from build123d import *

# Parameters (mm, degrees)
YAW_PLATFORM_START                         = 72
YAW_PLATFORM_PROFILE_R                     = 44
YAW_PLATFORM_DEPTH                         = 5
PRINTED_HOLLOW_YAW_SPINDLE_START           = 43
PRINTED_HOLLOW_YAW_SPINDLE_PROFILE_R       = 3.95
PRINTED_HOLLOW_YAW_SPINDLE_PROFILE_R_2     = 1.75
PRINTED_HOLLOW_YAW_SPINDLE_DEPTH           = 29
INNER_RACE_LOAD_SHOULDER_START             = 70
INNER_RACE_LOAD_SHOULDER_PROFILE_R         = 6
INNER_RACE_LOAD_SHOULDER_PROFILE_R_2       = 1.75
INNER_RACE_LOAD_SHOULDER_DEPTH             = 2
D_FLAT_ON_SPINDLE_END_START                = 43
D_FLAT_DRIVE_KEY_PROFILE_W                 = 3
D_FLAT_DRIVE_KEY_PROFILE_H                 = 10
D_FLAT_ON_SPINDLE_END_DEPTH                = 5
SHOULDER_MOUNT_PLATE_PROFILE_W             = 87
SHOULDER_MOUNT_PLATE_PROFILE_H             = 68
SHOULDER_MOUNT_PLATE_DEPTH                 = 4
MG996_BODY_WINDOW_START                    = -5
MG996_BODY_WINDOW_PROFILE_W                = 41.7
MG996_BODY_WINDOW_PROFILE_H                = 20.7
MG996_BODY_WINDOW_DEPTH                    = 162.869372409
MG996_TAB_MOUNTS_START                     = -50
MG996_TAB_MOUNTS_PROFILE_R                 = 1.9
MG996_TAB_MOUNTS_DEPTH                     = 207.869372409
PASSIVE_SHOULDER_STANDOFFS_START           = -50
PASSIVE_SHOULDER_STANDOFFS_PROFILE_R       = 1.6
PASSIVE_SHOULDER_STANDOFFS_DEPTH           = 207.869372409
UPRIGHT_RIB_START                          = -8
UPRIGHT_RIB_PROFILE_W                      = 7
UPRIGHT_RIB_PROFILE_H                      = 31
UPRIGHT_RIB_DEPTH                          = 12
YAW_POSITIVE_RETENTION_CROSSBOLT_START     = -10
YAW_POSITIVE_RETENTION_CROSSBOLT_PROFILE_R = 1.1
YAW_POSITIVE_RETENTION_CROSSBOLT_DEPTH     = 167.869372409


with BuildPart() as part:
    # Yaw_platform_profile → Yaw_platform (new body)
    with BuildSketch(Plane(origin=(0, 0, 0), x_dir=(1, 0, 0), z_dir=(0, 1, 0)).offset(YAW_PLATFORM_START)):
        with Locations(Location((0, 0, 0), (0, 0, 270))):
            Circle(YAW_PLATFORM_PROFILE_R)
    extrude(amount=YAW_PLATFORM_DEPTH)

    # Printed_hollow_yaw_spindle_profile → Printed_hollow_yaw_spindle (add)
    with BuildSketch(Plane(origin=(0, 0, 0), x_dir=(1, 0, 0), z_dir=(0, 1, 0)).offset(PRINTED_HOLLOW_YAW_SPINDLE_START)):
        with Locations(Location((0, 0, 0), (0, 0, 90))):
            Circle(PRINTED_HOLLOW_YAW_SPINDLE_PROFILE_R)
        with Locations(Location((0, 0, 0), (0, 0, 90))):
            Circle(PRINTED_HOLLOW_YAW_SPINDLE_PROFILE_R_2, mode=Mode.SUBTRACT)
    extrude(amount=PRINTED_HOLLOW_YAW_SPINDLE_DEPTH)

    # Inner_race_load_shoulder_profile → Inner_race_load_shoulder (add)
    with BuildSketch(Plane(origin=(0, 0, 0), x_dir=(1, 0, 0), z_dir=(0, 1, 0)).offset(INNER_RACE_LOAD_SHOULDER_START)):
        with Locations(Location((0, 0, 0), (0, 0, 270))):
            Circle(INNER_RACE_LOAD_SHOULDER_PROFILE_R)
        with Locations(Location((0, 0, 0), (0, 0, 90))):
            Circle(INNER_RACE_LOAD_SHOULDER_PROFILE_R_2, mode=Mode.SUBTRACT)
    extrude(amount=INNER_RACE_LOAD_SHOULDER_DEPTH)

    # D_flat_drive_key_profile → D_flat_on_spindle_end (cut)
    with BuildSketch(Plane(origin=(0, 0, 0), x_dir=(1, 0, 0), z_dir=(0, 1, 0)).offset(D_FLAT_ON_SPINDLE_END_START)):
        with Locations((4.5, 0)):
            Rectangle(D_FLAT_DRIVE_KEY_PROFILE_W, D_FLAT_DRIVE_KEY_PROFILE_H)
    extrude(amount=D_FLAT_ON_SPINDLE_END_DEPTH, mode=Mode.SUBTRACT)

    # Shoulder_mount_plate_profile → Shoulder_mount_plate (add)
    with BuildSketch(Plane.XY):
        with Locations((-0.5, 110)):
            Rectangle(SHOULDER_MOUNT_PLATE_PROFILE_W, SHOULDER_MOUNT_PLATE_PROFILE_H)
    extrude(amount=SHOULDER_MOUNT_PLATE_DEPTH)

    # MG996_body_window_profile → MG996_body_window (cut, through all)
    with BuildSketch(Plane.XY.offset(MG996_BODY_WINDOW_START)):
        with Locations((10.35, 122)):
            Rectangle(MG996_BODY_WINDOW_PROFILE_W, MG996_BODY_WINDOW_PROFILE_H)
    extrude(amount=MG996_BODY_WINDOW_DEPTH, mode=Mode.SUBTRACT)

    # MG996_tab_mounts_profile → MG996_tab_mounts (cut, through all)
    with BuildSketch(Plane.XY.offset(MG996_TAB_MOUNTS_START)):
        with Locations(Location((-13, 117, 0), (0, 0, 180))):
            Circle(MG996_TAB_MOUNTS_PROFILE_R)
        with Locations(Location((-13, 127, 0), (0, 0, 180))):
            Circle(MG996_TAB_MOUNTS_PROFILE_R)
        with Locations(Location((34, 117, 0), (0, 0, 180))):
            Circle(MG996_TAB_MOUNTS_PROFILE_R)
        with Locations(Location((34, 127, 0), (0, 0, 180))):
            Circle(MG996_TAB_MOUNTS_PROFILE_R)
    extrude(amount=MG996_TAB_MOUNTS_DEPTH, mode=Mode.SUBTRACT)

    # Passive_shoulder_standoffs_profile → Passive_shoulder_standoffs (cut, through all)
    with BuildSketch(Plane.XY.offset(PASSIVE_SHOULDER_STANDOFFS_START)):
        with Locations(Location((-36, 104, 0), (0, 0, 180))):
            Circle(PASSIVE_SHOULDER_STANDOFFS_PROFILE_R)
        with Locations(Location((-36, 140, 0), (0, 0, 180))):
            Circle(PASSIVE_SHOULDER_STANDOFFS_PROFILE_R)
    extrude(amount=PASSIVE_SHOULDER_STANDOFFS_DEPTH, mode=Mode.SUBTRACT)

    # Upright_rib_profile → Upright_rib (add)
    with BuildSketch(Plane.XY.offset(UPRIGHT_RIB_START)):
        with Locations((-19.5, 92.5)):
            Rectangle(UPRIGHT_RIB_PROFILE_W, UPRIGHT_RIB_PROFILE_H)
    extrude(amount=UPRIGHT_RIB_DEPTH)

    # Yaw_positive_retention_crossbolt_profile → Yaw_positive_retention_crossbolt (cut, through all)
    with BuildSketch(Plane(origin=(0, 0, 0), x_dir=(0, 0, -1), z_dir=(1, 0, 0)).offset(YAW_POSITIVE_RETENTION_CROSSBOLT_START)):
        with Locations(Location((0, 45.5, 0), (0, 0, 180))):
            Circle(YAW_POSITIVE_RETENTION_CROSSBOLT_PROFILE_R)
    extrude(amount=YAW_POSITIVE_RETENTION_CROSSBOLT_DEPTH, mode=Mode.SUBTRACT)


solid = part.part
Could you check a few things on this model? Use its own coordinates, in mm. A direction names the side the tool comes from. Coordinates: 2 decimals unless noted, no trailing zeros. Loops run counter-clockwise (first coordinate to the right, second up) from the corner with the lowest first, then second, coordinate; pieces in that order, holes last.
1. Imagine slicing it at D-D (x = -13.5). Please give me the cut outline in (y, z), and give its area (3 significant figures).
2. For P1, Ø10, axis at x = -25, y = 64, coming from the -Z side; P2, Ø12, axis at x = -21.5, z = -17.5, coming from the +Y side; P3, Ø2.5, axis at y = 45.5, z = 0, coming from the -X side; P4, Ø1, axis at x = 23.5, z = 16, coming from the -Y side, each with a flat end and sliding along its axis, tell me the tip position at first contact or that it passes through.
3. We'd pull the mould along Y, two halves only. Please class faces 1 (the face through (-9, 72, -1)), 2 (the face through (10, 132.35, 2)), 3 (the face through (-44, 110, 2)): released by +Y, released by -Y, zero draft, split by the parting line, or undercut.
4. For faces 4 (the face through (3, 44, 0)), 5 (the face through (-3.916, 56.311, 0.514)), 6 (the face through (-20, 108, -4)), which set-ups out of +Z, -Z, +X, -X, +Y, -Y let a thin tool reach every point of the face, with its end or its side?
5. Imagine slicing it at B-B (y = 127). Please give me the cut outline in (x, z), and give its area (3 significant figures).
6. Imagine slicing it at A-A (x = 0). Please give me the cut outline in (y, z), and give its area (3 significant figures).
7. I need wall thicknesses on L1, parallel to Y at x = -13, z = 1; L2, parallel to X at y = 127, z = 1.55; L3, parallel to Y at x = 25.5, z = 9.5. Which ranges of each line are inside material? Lowest first, please.
8. Imagine slicing it at C-C (y = 140). Please give me the cut outline in (x, z).
Computed values:
1. outline: (72, -41.88) - (77, -41.88) - (77, 0) - (115.17, 0) - (115.17, 4) - (77, 4) - (77, 41.88) - (72, 41.88) - close; (118.83, 0) - (125.17, 0) - (125.17, 4) - (118.83, 4) - close; (128.83, 0) - (144, 0) - (144, 4) - (128.83, 4) - close
1. area: 657 mm2
2. P1: passes through
2. P2: stops at y = 77
2. P3: stops at x = -3.95
2. P4: stops at y = 72
3. face 1: released by -Y
3. face 2: undercut
3. face 3: zero draft
4. face 4: +Z, -Z, +X, -Y
4. face 5: -Y
4. face 6: -Z, +X, -X, +Y
5. outline: (-44, 0) - (-14.9, 0) - (-14.9, 4) - (-44, 4) - close; (-11.1, 0) - (-10.5, 0) - (-10.5, 4) - (-11.1, 4) - close; (31.2, 0) - (32.1, 0) - (32.1, 4) - (31.2, 4) - close; (35.9, 0) - (43, 0) - (43, 4) - (35.9, 4) - close
5. area: 151 mm2
6. outline: (43, -3.95) - (70, -3.95) - (70, -6) - (72, -6) - (72, -44) - (77, -44) - (77, 0) - (111.65, 0) - (111.65, 4) - (77, 4) - (77, 44) - (72, 44) - (72, 6) - (70, 6) - (70, 3.95) - (43, 3.95) - (43, 1.75) - (72, 1.75) - (72, -1.75) - (43, -1.75) - close; (132.35, 0) - (144, 0) - (144, 4) - (132.35, 4) - close
6. area: 761 mm2
7. L1: y = 72 to 115.1, 118.9 to 125.1, 128.9 to 144
7. L2: x = -44 to -14.9, -11.1 to -10.5, 31.2 to 32.1, 35.9 to 43
7. L3: y = 72 to 77
8. outline: (-44, 0) - (-37.6, 0) - (-37.6, 4) - (-44, 4) - close; (-34.4, 0) - (43, 0) - (43, 4) - (-34.4, 4) - close
